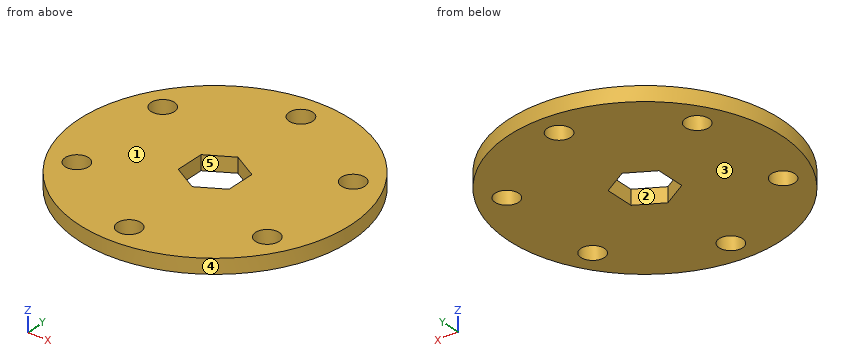
Autodesk Inventor part; units mm, degrees
ref_plane "YZ Plane" through (0, 0, 0) normal (1, 0, 0) x (0, 1, 0)
ref_plane "XZ Plane" through (0, 0, 0) normal (0, 1, 0) x (-1, 0, 0)
ref_plane "XY Plane" through (0, 0, 0) normal (0, 0, 1) x (1, 0, 0)
sketch "Sketch1" plane through (0, 0, 0) normal (0, 0, 1) x (1, 0, 0)
  arc A0 (24.3719, -16.0061) -> (18.9457, -6.6082) centre (20.6227, -11.9054) ccw
  arc A1 (18.9457, -6.6082) -> (15.375, -3.3543) centre (0, -23.8125) ccw
  arc A2 (15.4859, -6.1082) -> (15.375, -3.3543) centre (14.3062, -4.7765) ccw
  arc A3 (15.4859, -6.1082) -> (13.3187, -9.3259) centre (20.6222, -11.9062) ccw
  arc A4 (10.5541, -10.1415) -> (13.3187, -9.3259) centre (11.6413, -8.7333) ccw
  arc A5 (10.5541, -10.1415) -> (6.5626, -7.8369) centre (0, -23.8125) ccw
  arc A6 (5.8865, -5.0351) -> (6.5626, -7.8369) centre (7.2386, -6.1913) ccw
  arc A7 (5.8865, -5.0351) -> (7.5891, -1.5492) centre (-0.0005, -0.0009) ccw
  arc A8 (10.0295, -0.2681) -> (7.5891, -1.5492) centre (9.3323, -1.9049) ccw
  arc A9 (10.0295, -0.2681) -> (5.4257, 1.1973) centre (0, -23.8125) ccw
  arc A10 (5.4257, 1.1973) -> (-5.4257, 1.1973) centre (0, 0) ccw
  arc A11 (-5.4257, 1.1973) -> (-10.0298, -0.2683) centre (0, -23.8125) ccw
  arc A12 (-7.5894, -1.5492) -> (-10.0298, -0.2683) centre (-9.3326, -1.905) ccw
  arc A13 (-7.5894, -1.5492) -> (-5.8864, -5.0349) centre (0, 0) ccw
  arc A14 (-6.5624, -7.8369) -> (-5.8864, -5.0349) centre (-7.2384, -6.1912) ccw
  arc A15 (-6.5624, -7.8369) -> (-10.554, -10.1414) centre (0, -23.8125) ccw
  arc A16 (-13.3185, -9.326) -> (-10.554, -10.1414) centre (-11.6411, -8.7331) ccw
  arc A17 (-13.3185, -9.326) -> (-15.486, -6.1085) centre (-20.6217, -11.9071) ccw
  arc A18 (-15.3753, -3.3545) -> (-15.486, -6.1085) centre (-14.3064, -4.7767) ccw
  arc A19 (-15.3753, -3.3545) -> (-18.9467, -6.6093) centre (0, -23.8125) ccw
  arc A20 (-18.9467, -6.6093) -> (-24.3721, -16.0067) centre (-20.6217, -11.9071) ccw
  arc A21 (-24.3721, -16.0067) -> (-25.4048, -20.7264) centre (0, -23.8125) ccw
  arc A22 (-23.0753, -19.2535) -> (-25.4048, -20.7264) centre (-23.6387, -20.941) ccw
  arc A23 (-23.0753, -19.2535) -> (-19.2051, -19.5215) centre (-20.6222, -11.9063) ccw
  arc A24 (-17.1165, -21.5079) -> (-19.2051, -19.5215) centre (-18.8796, -21.2705) ccw
  arc A25 (-17.1165, -21.5079) -> (-17.1165, -26.1169) centre (0, -23.8125) ccw
  arc A26 (-19.2049, -28.1034) -> (-17.1165, -26.1169) centre (-18.8797, -26.3543) ccw
  arc A27 (-19.2049, -28.1034) -> (-23.0751, -28.3718) centre (-20.6212, -35.7187) ccw
  arc A28 (-25.4048, -26.8989) -> (-23.0751, -28.3718) centre (-23.6387, -26.6843) ccw
  arc A29 (-25.4048, -26.8989) -> (-24.3714, -31.6203) centre (0, -23.8125) ccw
  arc A30 (-24.3714, -31.6203) -> (-18.9453, -41.0172) centre (-20.6207, -35.7196) ccw
  arc A31 (-18.9453, -41.0172) -> (-15.375, -44.2707) centre (0, -23.8125) ccw
  arc A32 (-15.4859, -41.5168) -> (-15.375, -44.2707) centre (-14.3062, -42.8485) ccw
  arc A33 (-15.4859, -41.5168) -> (-13.3187, -38.2991) centre (-20.6222, -35.7188) ccw
  arc A34 (-10.5541, -37.4835) -> (-13.3187, -38.2991) centre (-11.6413, -38.8917) ccw
  arc A35 (-10.5541, -37.4835) -> (-6.5626, -39.7881) centre (0, -23.8125) ccw
  arc A36 (-5.8865, -42.5899) -> (-6.5626, -39.7881) centre (-7.2386, -41.4337) ccw
  arc A37 (-5.8865, -42.5899) -> (-7.5891, -46.0758) centre (0.0005, -47.6241) ccw
  arc A38 (-10.0295, -47.3569) -> (-7.5891, -46.0758) centre (-9.3323, -45.7201) ccw
  arc A39 (-10.0295, -47.3569) -> (-5.4236, -48.8227) centre (0, -23.8125) ccw
  arc A40 (-5.4236, -48.8227) -> (5.4278, -48.8218) centre (0.002, -47.625) ccw
  arc A41 (5.4278, -48.8218) -> (10.0298, -47.3567) centre (0, -23.8125) ccw
  arc A42 (7.5894, -46.0758) -> (10.0298, -47.3567) centre (9.3326, -45.72) ccw
  arc A43 (7.5894, -46.0758) -> (5.8864, -42.5901) centre (0, -47.625) ccw
  arc A44 (6.5624, -39.7881) -> (5.8864, -42.5901) centre (7.2384, -41.4338) ccw
  arc A45 (6.5624, -39.7881) -> (10.554, -37.4836) centre (0, -23.8125) ccw
  arc A46 (13.3185, -38.299) -> (10.554, -37.4836) centre (11.6411, -38.8919) ccw
  arc A47 (13.3185, -38.299) -> (15.486, -41.5165) centre (20.6217, -35.7179) ccw
  arc A48 (15.3753, -44.2705) -> (15.486, -41.5165) centre (14.3064, -42.8483) ccw
  arc A49 (15.3753, -44.2705) -> (18.9472, -41.0152) centre (0, -23.8125) ccw
  arc A50 (18.9472, -41.0152) -> (24.3725, -31.6169) centre (20.6237, -35.7179) ccw
  arc A51 (24.3725, -31.6169) -> (25.4048, -26.8986) centre (0, -23.8125) ccw
  arc A52 (23.0753, -28.3715) -> (25.4048, -26.8986) centre (23.6387, -26.684) ccw
  arc A53 (23.0753, -28.3715) -> (19.2051, -28.1035) centre (20.6222, -35.7187) ccw
  arc A54 (17.1165, -26.1171) -> (19.2051, -28.1035) centre (18.8796, -26.3545) ccw
  arc A55 (17.1165, -26.1171) -> (17.1165, -21.5081) centre (0, -23.8125) ccw
  arc A56 (19.2049, -19.5216) -> (17.1165, -21.5081) centre (18.8797, -21.2707) ccw
  arc A57 (19.2049, -19.5216) -> (23.0751, -19.2532) centre (20.6212, -11.9063) ccw
  arc A58 (25.4048, -20.7261) -> (23.0751, -19.2532) centre (23.6387, -20.9407) ccw
  arc A59 (25.4048, -20.7261) -> (24.3719, -16.0061) centre (0, -23.8125) ccw
  circle A60 centre (20.6227, -11.9054) radius 2.54
  circle A61 centre (20.6237, -35.7179) radius 2.54
  circle A62 centre (0.002, -47.625) radius 2.54
  circle A63 centre (-20.6207, -35.7196) radius 2.54
  circle A64 centre (-20.6217, -11.9071) radius 2.54
  circle A65 centre (0, 0) radius 2.54
  circle A66 centre (0, -23.8125) radius 14.2875
  circle A67 centre (0, -23.8125) radius 29.3688
  circle A68 centre (0, -23.8125) radius 6.35
  line L0 (0, 0) -> (0, -17.4625)
  line L1 (20.6227, -11.9054) -> (5.4278, -20.5169)
  line L2 (0, -17.4625) -> (5.4993, -20.6375)
  line L3 (5.4993, -20.6375) -> (5.4993, -26.9875)
  line L4 (5.4993, -26.9875) -> (0, -30.1625)
  line L5 (0, -30.1625) -> (-5.4993, -26.9875)
  line L6 (-5.4993, -26.9875) -> (-5.4993, -20.6375)
  line L7 (-5.4993, -20.6375) -> (0, -17.4625)
  dimension "d0" = 12.7
extrude "Extrusion1" add sketch "Sketch1" along normal blind 3.175 contours A59 A58 A57 A56 A55 A54 A53 A52 A51 A50 A49 A48 A47 A46 A45 A44 A43 A42 A41 A40 A39 A38 A37 A36 A35 A34 A33 A32 A31 A30 A29 A28 A27 A26 A25 A24 A23 A22 A21 A20 A19 A18 A17 A16 A15 A14 A13 A12 A11 A10 A9 A8 A7 A6 A5 A4 A3 A2 A1 A0 | A0 A67 A50 A51 A52 A53 A54 A55 A56 A57 A58 A59 | A0 A1 A2 A3 A4 A5 A6 A7 A8 A9 A10 A67 | A10 A11 A12 A13 A14 A15 A16 A17 A18 A19 A20 A67 | A67 A40 A41 A42 A43 A44 A45 A46 A47 A48 A49 A50 | A20 A21 A22 A23 A24 A25 A26 A27 A28 A29 A30 A67 | A67 A30 A31 A32 A33 A34 A35 A36 A37 A38 A39 A40 | A66 L0 A68 L1 | L1 A68 L0 A66 | A68 L2 | L7 A68 | A68 L3 | L6 A68 | A68 L4 | L5 A68
properties part number "wheelhubthing" material "Aluminum 6061"
Design review of the part built by this model. Coordinates are the model's own, in mm. Face numbers are marked on the shaded views. A direction names the side the tool comes from. Coordinates: 2 decimals unless noted, no trailing zeros. Loops run counter-clockwise (first coordinate to the right, second up) from the corner with the lowest first, then second, coordinate; pieces in that order, holes last. Notation, with made-up numbers: (58, -34) -> (71, -34) arc R24 ccw to (71, 4) -> close; hole circle Ø5 at (-15.5, 7). An arc over 180 degrees is marked (long way). Answer as a JSON object with one key per item and string values.
Q1. The part is to be moulded in two halves that separate along Y. For the marked faces 3, 4 and 5, say which applies: +Y half, -Y half, draft (parallel to the pull), parting line (faces both ways), or undercut.
Answer block:
{"face 3": "draft", "face 4": "parting line", "face 5": "undercut"}
Q2. Take a section at B-B on z = 2.1. Give the boundary of the cut face in (x, y) (1 decimal), plus the area to 3 significant figures.
Answer block:
{"outline": "circle Ø58.7 at (0, -23.8); hole circle Ø5.1 at (-20.6, -35.7); hole circle Ø5.1 at (-20.6, -11.9); hole (-5.5, -27) -> (0, -30.2) -> (5.5, -27) -> (5.5, -20.6) -> (0, -17.5) -> (-5.5, -20.6) -> close; hole circle Ø5.1 at (0, -47.6); hole circle Ø5.1 at (0, 0); hole circle Ø5.1 at (20.6, -35.7); hole circle Ø5.1 at (20.6, -11.9)", "area": "2,480 mm^2"}
Q3. To check wall thickness, follow L1, parallel to Y at x = -19.5, z = 2.45; L2, parallel to Y at x = 22.5, z = 1.95; L3, parallel to X at y = -23.5, z = 1.9. State the ranges of each line that lie inside material, in increasing order.
Answer block:
{"L1": "y = -45.77 to -38, -33.44 to -14.19, -9.63 to -1.85", "L2": "y = -42.69 to -37.43, -34.01 to -13.62, -10.19 to -4.94", "L3": "x = -29.37 to -5.5, 5.5 to 29.37"}
Q4. Take a section at D-D on x = 8. Give the boundary of the cut face in (y, z) (3 decimals), plus the area to 3 significant figures.
Answer block:
{"outline": "(-52.071, 0) -> (4.446, 0) -> (4.446, 3.175) -> (-52.071, 3.175) -> close", "area": "179 mm^2"}
Q5. Take a section at A-A on y = -49. Give the boundary of the cut face in (x, z) (3 decimals), plus the area to 3 significant figures.
Answer block:
{"outline": "(-15.104, 0) -> (-2.134, 0) -> (-2.134, 3.175) -> (-15.104, 3.175) -> close; (2.138, 0) -> (15.104, 0) -> (15.104, 3.175) -> (2.138, 3.175) -> close", "area": "82.3 mm^2"}
Q6. Tool access review of the marked faces 1 and 2: name each direction out of +Z, -Z, +X, -X, +Y, -Y from which nothing blocks a thin tool from reaching the whole face with its end or side.
Answer block:
{"face 1": "+Z, +X, -X, +Y, -Y", "face 2": "+Z, -Z"}
Q7. Clearance check with flat-ended pins moving along their axes: pin 1 Ø1 at (y, z) = (-40.5, 0.5) entering from -X; pin 2 Ø1 at (y, z) = (-42.5, 2) entering from -X; pin 3 Ø3 at (x, y) = (-20.62, -11.91) entering from -Z; pin 4 Ø1 at (y, z) = (-23, 1) entering from +X. State where each tip first meets the part, or that it passes through.
Answer block:
{"pin 1": "stops at x = -24.5", "pin 2": "stops at x = -23.06", "pin 3": "passes through", "pin 4": "stops at x = 29.37"}
Q8. Take a section at C-C on y = -21.5. Give the boundary of the cut face in (x, z) (3 decimals), plus the area to 3 significant figures.
Answer block:
{"outline": "(-29.278, 0) -> (-5.499, 0) -> (-5.499, 3.175) -> (-29.278, 3.175) -> close; (5.499, 0) -> (29.278, 0) -> (29.278, 3.175) -> (5.499, 3.175) -> close", "area": "151 mm^2"}
